```python
from build123d import *

# Parameters (mm, degrees)
SKETCH_2_W           = 80
SKETCH_2_H           = 34
SKETCH_2_R           = 4.05
EXTRUDE_1_DEPTH      = 8
SKETCH_3_R           = 2.55
CUT_EXTRUDE_1_DEPTH  = 88.292611371
CUT_EXTRUDE_2_DEPTH  = 88.292611371
SKETCH_5_R           = 1.55
CUT_EXTRUDE_3_DEPTH  = 88.292611371
CUT_EXTRUDE_4_DEPTH  = 6
CUT_EXTRUDE_5_DEPTH  = 4.5
SKETCH_25_R          = 1.55
CUT_EXTRUDE_13_DEPTH = 88.292611371
CUT_EXTRUDE_11_DEPTH = 2
EXTRUDE_2_DEPTH      = 8
SKETCH_26_R          = 5.5
CUT_EXTRUDE_14_DEPTH = 89.926936302


with BuildPart() as part:
    # 草图2 → 凸台-拉伸1 (new body)
    with BuildSketch(Plane.XY):
        with Locations((40, 17)):
            Rectangle(SKETCH_2_W, SKETCH_2_H)
        with Locations((7, 8)):
            Circle(SKETCH_2_R, mode=Mode.SUBTRACT)
        with Locations((40, 10)):
            Circle(SKETCH_2_R, mode=Mode.SUBTRACT)
        with Locations((73, 8)):
            Circle(SKETCH_2_R, mode=Mode.SUBTRACT)
    extrude_1 = extrude(amount=EXTRUDE_1_DEPTH)

    # 草图3 → 切除-拉伸1 (cut, through all)
    with BuildSketch(Plane.XY.offset(8)):
        with Locations((23, 8)):
            Circle(SKETCH_3_R)
        with Locations((57, 8)):
            Circle(SKETCH_3_R)
    extrude(amount=-CUT_EXTRUDE_1_DEPTH, mode=Mode.SUBTRACT)

    # 草图4 → 切除-拉伸2 (cut, through all)
    with BuildSketch(Plane(origin=(80, 0, 0), x_dir=(0, 0, -1), z_dir=(1, 0, 0))):
        Polygon((-1.5, 32.2), (-2.5, 32.2), (-2.5, 34), (0, 34), (0, 28.8), (-1.5, 28.8), align=None)
    cut_extrude_2 = extrude(amount=-CUT_EXTRUDE_2_DEPTH, mode=Mode.SUBTRACT)

    # 草图5 → 切除-拉伸3 (cut, through all)
    with BuildSketch(Plane.XY.offset(8)):
        with Locations((48, 10)):
            Circle(SKETCH_5_R)
        with Locations((32, 10)):
            Circle(SKETCH_5_R)
    cut_extrude_3 = extrude(amount=-CUT_EXTRUDE_3_DEPTH, mode=Mode.SUBTRACT)

    # 草图7 → 切除-拉伸4 (cut)
    with BuildSketch(Plane(origin=(0, 0, 0), x_dir=(-1, 0, 0), z_dir=(0, 0, -1))):
        Polygon((-52.9, 5.632863896), (-52.9, 10.367136104), (-57, 12.734272207), (-61.1, 10.367136104), (-61.1, 5.632863896), (-57, 3.265727793), align=None)
        Polygon((-27.1, 5.632863896), (-23, 3.265727793), (-18.9, 5.632863896), (-18.9, 10.367136104), (-23, 12.734272207), (-27.1, 10.367136104), align=None)
    extrude(amount=-CUT_EXTRUDE_4_DEPTH, mode=Mode.SUBTRACT)

    # 草图8 → 切除-拉伸5 (cut)
    with BuildSketch(Plane(origin=(0, 0, 0), x_dir=(-1, 0, 0), z_dir=(0, 0, -1))):
        Polygon((-48, 6.709103466), (-45.15, 8.354551733), (-45.15, 11.645448267), (-48, 13.290896534), (-50.85, 11.645448267), (-50.85, 8.354551733), align=None)
        Polygon((-32, 6.709103466), (-29.15, 8.354551733), (-29.15, 11.645448267), (-32, 13.290896534), (-34.85, 11.645448267), (-34.85, 8.354551733), align=None)
    cut_extrude_5 = extrude(amount=-CUT_EXTRUDE_5_DEPTH, mode=Mode.SUBTRACT)

    # 草图25 → 切除-拉伸13 (cut, through all)
    with BuildSketch(Plane(origin=(0, 0, 0), x_dir=(-1, 0, 0), z_dir=(0, 0, -1))):
        with Locations((-60, 25)):
            Circle(SKETCH_25_R)
        with Locations((-20, 25)):
            Circle(SKETCH_25_R)
    cut_extrude_13 = extrude(amount=-CUT_EXTRUDE_13_DEPTH, mode=Mode.SUBTRACT)

    # 草图19 → 切除-拉伸11 (cut)
    with BuildSketch(Plane(origin=(0, 0, 2.5), x_dir=(-1, 0, 0), z_dir=(0, 0, -1))):
        with BuildLine():
            Line((-25, 34), (-55.247938178, 34))
            Line((-55.247938178, 34), (-55.247938178, 33.2))
            ThreePointArc((-55.247938178, 33.2), (-54.747938178, 32.7), (-54.247938178, 33.2))
            Line((-54.247938178, 33.2), (-26, 33.2))
            ThreePointArc((-26, 33.2), (-25.5, 32.7), (-25, 33.2))
            Line((-25, 33.2), (-25, 34))
        make_face()
    cut_extrude_11 = extrude(amount=-CUT_EXTRUDE_11_DEPTH, mode=Mode.SUBTRACT)

    # 草图22 → 凸台-拉伸2 (add)
    with BuildSketch(Plane.XY.offset(8)):
        with BuildLine():
            Line((0, -4), (5.5, -4))
            ThreePointArc((5.5, -4), (3.5, -2), (5.5, 0))
            Line((5.5, 0), (0, 0))
            ThreePointArc((0, 0), (2, -2), (0, -4))
        make_face()
        with BuildLine():
            Line((80, 0), (74.5, 0))
            ThreePointArc((74.5, 0), (76.5, -2), (74.5, -4))
            Line((74.5, -4), (80, -4))
            ThreePointArc((80, -4), (78, -2), (80, 0))
        make_face()
    extrude(amount=-EXTRUDE_2_DEPTH)

    # 镜向2: 凸台-拉伸1, 切除-拉伸2, 切除-拉伸3, 切除-拉伸5, 切除-拉伸13, 切除-拉伸11 across plane
    add(extrude_1.mirror(Plane(origin=(0, -2, 0), x_dir=(0, 0, 1), z_dir=(0, -1, 0))))
    add(cut_extrude_2.mirror(Plane(origin=(0, -2, 0), x_dir=(0, 0, 1), z_dir=(0, -1, 0))), mode=Mode.SUBTRACT)
    add(cut_extrude_3.mirror(Plane(origin=(0, -2, 0), x_dir=(0, 0, 1), z_dir=(0, -1, 0))), mode=Mode.SUBTRACT)
    add(cut_extrude_5.mirror(Plane(origin=(0, -2, 0), x_dir=(0, 0, 1), z_dir=(0, -1, 0))), mode=Mode.SUBTRACT)
    add(cut_extrude_13.mirror(Plane(origin=(0, -2, 0), x_dir=(0, 0, 1), z_dir=(0, -1, 0))), mode=Mode.SUBTRACT)
    add(cut_extrude_11.mirror(Plane(origin=(0, -2, 0), x_dir=(0, 0, 1), z_dir=(0, -1, 0))), mode=Mode.SUBTRACT)

    # 草图26 → 切除-拉伸14 (cut, through all)
    with BuildSketch(Plane(origin=(0, 0, 0), x_dir=(-1, 0, 0), z_dir=(0, 0, -1))):
        with Locations((-40, -14)):
            Circle(SKETCH_26_R)
    extrude(amount=-CUT_EXTRUDE_14_DEPTH, mode=Mode.SUBTRACT)


solid = part.part
```
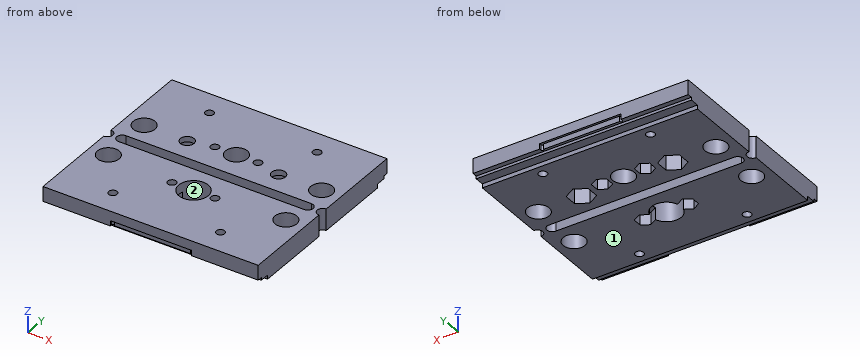
The listing builds one solid part. Answer for the finished solid, in the listing's coordinates (mm). Face numbers are marked on the shaded views. Round coordinates to 2 decimals unless told otherwise and drop trailing zeros. Loops run counter-clockwise (first coordinate to the right, second up) from the corner with the lowest first, then second, coordinate; pieces in that order, holes last.
1) Consider line 1 (X direction, y = -29, z = 2); line 2 (Y direction, x = 32, z = 5.25); line 3 (Y direction, x = 57, z = 7.65). Determine where each line is inside the solid, lowest interval first.
Outcome:
line 1: x = 0 to 18.45, 21.55 to 58.45, 61.55 to 80
line 2: y = -38 to -15.55, -12.45 to -4, 0 to 8.45, 11.55 to 34
line 3: y = -38 to -4, 0 to 5.45, 10.55 to 34
2) Given P1, Ø8, axis at x = 57, y = 8, coming from the -Z side; P2, Ø2.5, axis at x = 20, y = -29, coming from the +Z side; P3, Ø2, axis at x = 26, y = 32.5, coming from the -Z side; P4, Ø1, axis at x = 34, z = 3, coming from the +Y side, each flat-ended and moving along its own axis, determine where each tip first touches the part or whether it passes through.
Outcome:
P1: stops at z = 6
P2: passes through
P3: stops at z = 1.5
P4: stops at y = 33.2
3) A cutting plane is placed at B-B on x = 66.5. Determine the outline of the cut face in (y, z).
Outcome:
outline: (-38, 2.5) - (-36.2, 2.5) - (-36.2, 1.5) - (-32.8, 1.5) - (-32.8, 0) - (-4, 0) - (-4, 8) - (-38, 8) - close; (0, 0) - (28.8, 0) - (28.8, 1.5) - (32.2, 1.5) - (32.2, 2.5) - (34, 2.5) - (34, 8) - (0, 8) - close
4) A cutting plane is placed at A-A on x = 7. Determine the outline of the cut face in (y, z).
Outcome:
outline: (-38, 2.5) - (-36.2, 2.5) - (-36.2, 1.5) - (-32.8, 1.5) - (-32.8, 0) - (-16.05, 0) - (-16.05, 8) - (-38, 8) - close; (-7.95, 0) - (-4, 0) - (-4, 8) - (-7.95, 8) - close; (0, 0) - (3.95, 0) - (3.95, 8) - (0, 8) - close; (12.05, 0) - (28.8, 0) - (28.8, 1.5) - (32.2, 1.5) - (32.2, 2.5) - (34, 2.5) - (34, 8) - (12.05, 8) - close
5) A cutting plane is placed at C-C on y = 25. Determine the outline of the cut face in (x, z).
Outcome:
outline: (0, 0) - (18.45, 0) - (18.45, 8) - (0, 8) - close; (21.55, 0) - (58.45, 0) - (58.45, 8) - (21.55, 8) - close; (61.55, 0) - (80, 0) - (80, 8) - (61.55, 8) - close
6) A cutting plane is placed at D-D on y = -2. Determine the outline of the cut face in (x, z).
Outcome:
outline: (2, 0) - (3.5, 0) - (3.5, 8) - (2, 8) - close; (76.5, 0) - (78, 0) - (78, 8) - (76.5, 8) - close
7) For a pull along Y with two mould halves and no side action, classify the marked faces 1 and 2 as released by +Y, released by -Y, zero draft, split by the parting line, or undercut.
Outcome:
face 1: zero draft
face 2: undercut
